Build history of the part. All positions in model axes, mm. Face numbers are marked on the shaded views. A direction names the side the tool comes from. Round coordinates to 2 decimals unless told otherwise and drop trailing zeros. Write each loop counter-clockwise with the first axis right and the second up, starting at its lowest first coordinate (ties: lowest second). Pieces come first, ordered by that corner, then holes.
1) Which spindle directions (+Z, -Z, +X, -X, +Y, -Y) get a long thin tool onto all of the face, cutting with end or side? Do the marked faces 4, 5 and 6. Say none if no direction does.
2) Flat gauge pins, fed straight in: pin 1 (1.5 mm diameter, centred on x = 24.5, z = 2, fed in from -Y); pin 2 (3 mm diameter, centred on y = 7, z = -4, fed in from -X); pin 3 (1.4 mm diameter, centred on x = 24, z = -1, fed in from +Y); pin 4 (2 mm diameter, centred on x = 2, y = 2.5, fed in from -Z). Where does each tip first touch, or does it go through?
3) Saw through at A-A (y = 0). Write the cut outline in (x, z).
4) Saw through at C-C (y = 5.5). Write the cut outline in (x, z).
5) Wall check: probe 1 along Z at (x, y) = (5, 0); probe 2 along Y at (x, z) = (-23, 5.25); probe 3 along Z at (x, y) = (-18, -3.75). Give the ranges that are in metal, low to high.
6) Pull direction Z, two halves, no side cores. Call the marked faces 1, 2 and 3: +Z half, -Z half, draft (parallel to the pull), parting line (faces both ways), or undercut.
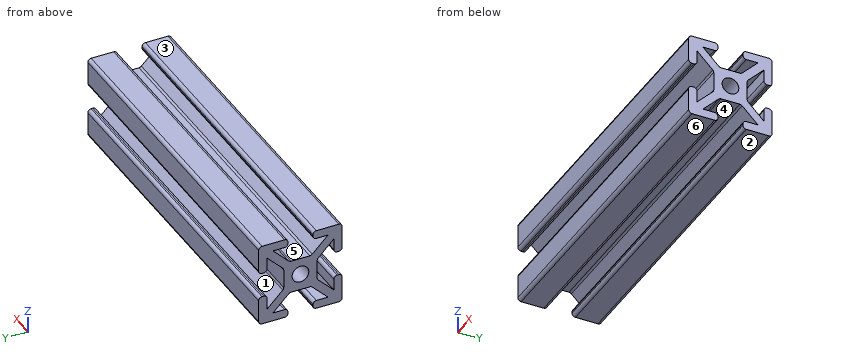
from build123d import *

# Parameters (mm, degrees)
SKETCH11_R          = 2
PROFILE_4X4_1_DEPTH = 80


with BuildPart() as part:
    # Sketch11 → Profile 4X4(1) (new body)
    with BuildSketch(Plane.YZ.offset(-35.597484277)):
        with BuildLine():
            Line((-3, 9.2), (-3, 8.8))
            ThreePointArc((-3, 8.8), (-3.234314575, 8.234314575), (-3.8, 8))
            Line((-3.8, 8), (-6.585786438, 8))
            Line((-6.585786438, 8), (-2.820101013, 4.234314575))
            ThreePointArc((-2.820101013, 4.234314575), (-2.560562334, 4.060896374), (-2.254415588, 4))
            Line((-2.254415588, 4), (2.254415588, 4))
            ThreePointArc((2.254415588, 4), (2.560562334, 4.060896374), (2.820101013, 4.234314575))
            Line((2.820101013, 4.234314575), (6.585786438, 8))
            Line((6.585786438, 8), (3.8, 8))
            ThreePointArc((3.8, 8), (3.234314575, 8.234314575), (3, 8.8))
            Line((3, 8.8), (3, 9.2))
            ThreePointArc((3, 9.2), (3.234314575, 9.765685425), (3.8, 10))
            Line((3.8, 10), (9.2, 10))
            ThreePointArc((9.2, 10), (9.765685425, 9.765685425), (10, 9.2))
            Line((10, 9.2), (10, 3.8))
            ThreePointArc((10, 3.8), (9.765685425, 3.234314575), (9.2, 3))
            Line((9.2, 3), (8.8, 3))
            ThreePointArc((8.8, 3), (8.234314575, 3.234314575), (8, 3.8))
            Line((8, 3.8), (8, 6.585786438))
            Line((8, 6.585786438), (4.234314575, 2.820101013))
            ThreePointArc((4.234314575, 2.820101013), (4.060896374, 2.560562334), (4, 2.254415588))
            Line((4, 2.254415588), (4, -2.254415588))
            ThreePointArc((4, -2.254415588), (4.060896374, -2.560562334), (4.234314575, -2.820101013))
            Line((4.234314575, -2.820101013), (8, -6.585786438))
            Line((8, -6.585786438), (8, -3.8))
            ThreePointArc((8, -3.8), (8.234314575, -3.234314575), (8.8, -3))
            Line((8.8, -3), (9.2, -3))
            ThreePointArc((9.2, -3), (9.765685425, -3.234314575), (10, -3.8))
            Line((10, -3.8), (10, -9.2))
            ThreePointArc((10, -9.2), (9.765685425, -9.765685425), (9.2, -10))
            Line((9.2, -10), (3.8, -10))
            ThreePointArc((3.8, -10), (3.234314575, -9.765685425), (3, -9.2))
            Line((3, -9.2), (3, -8.8))
            ThreePointArc((3, -8.8), (3.234314575, -8.234314575), (3.8, -8))
            Line((3.8, -8), (6.585786438, -8))
            Line((6.585786438, -8), (2.820101013, -4.234314575))
            ThreePointArc((2.820101013, -4.234314575), (2.560562334, -4.060896374), (2.254415588, -4))
            Line((2.254415588, -4), (-2.254415588, -4))
            ThreePointArc((-2.254415588, -4), (-2.560562334, -4.060896374), (-2.820101013, -4.234314575))
            Line((-2.820101013, -4.234314575), (-6.585786438, -8))
            Line((-6.585786438, -8), (-3.8, -8))
            ThreePointArc((-3.8, -8), (-3.234314575, -8.234314575), (-3, -8.8))
            Line((-3, -8.8), (-3, -9.2))
            ThreePointArc((-3, -9.2), (-3.234314575, -9.765685425), (-3.8, -10))
            Line((-3.8, -10), (-9.2, -10))
            ThreePointArc((-9.2, -10), (-9.765685425, -9.765685425), (-10, -9.2))
            Line((-10, -9.2), (-10, -3.8))
            ThreePointArc((-10, -3.8), (-9.765685425, -3.234314575), (-9.2, -3))
            Line((-9.2, -3), (-8.8, -3))
            ThreePointArc((-8.8, -3), (-8.234314575, -3.234314575), (-8, -3.8))
            Line((-8, -3.8), (-8, -6.585786438))
            Line((-8, -6.585786438), (-4.234314575, -2.820101013))
            ThreePointArc((-4.234314575, -2.820101013), (-4.060896374, -2.560562334), (-4, -2.254415588))
            Line((-4, -2.254415588), (-4, 2.254415588))
            ThreePointArc((-4, 2.254415588), (-4.060896374, 2.560562334), (-4.234314575, 2.820101013))
            Line((-4.234314575, 2.820101013), (-8, 6.585786438))
            Line((-8, 6.585786438), (-8, 3.8))
            ThreePointArc((-8, 3.8), (-8.234314575, 3.234314575), (-8.8, 3))
            Line((-8.8, 3), (-9.2, 3))
            ThreePointArc((-9.2, 3), (-9.765685425, 3.234314575), (-10, 3.8))
            Line((-10, 3.8), (-10, 9.2))
            ThreePointArc((-10, 9.2), (-9.765685425, 9.765685425), (-9.2, 10))
            Line((-9.2, 10), (-3.8, 10))
            ThreePointArc((-3.8, 10), (-3.234314575, 9.765685425), (-3, 9.2))
        make_face()
        Circle(SKETCH11_R, mode=Mode.SUBTRACT)
    extrude(amount=PROFILE_4X4_1_DEPTH)


solid = part.part
Evaluation:
1. face 4: -Z, +X, -X
1. face 5: +Z, +X, -X
1. face 6: -Z, +X, -X, +Y, -Y
2. pin 1: stops at y = -4.17
2. pin 2: stops at x = -35.6
2. pin 3: stops at y = 4
2. pin 4: stops at z = -9.94
3. outline: (-35.6, -4) - (44.4, -4) - (44.4, -2) - (-35.6, -2) - close; (-35.6, 2) - (44.4, 2) - (44.4, 4) - (-35.6, 4) - close
4. outline: (-35.6, -10) - (44.4, -10) - (44.4, -8) - (-35.6, -8) - close; (-35.6, -6.91) - (44.4, -6.91) - (44.4, -4.09) - (-35.6, -4.09) - close; (-35.6, 4.09) - (44.4, 4.09) - (44.4, 6.91) - (-35.6, 6.91) - close; (-35.6, 8) - (44.4, 8) - (44.4, 10) - (-35.6, 10) - close
5. probe 1: z = -4 to -2, 2 to 4
5. probe 2: y = -10 to -8, -6.66 to -3.84, 3.84 to 6.66, 8 to 10
5. probe 3: z = -10 to -8, -5.16 to 5.16, 8 to 10
6. face 1: undercut
6. face 2: -Z half
6. face 3: +Z half
